Input: part model. Units: mm. Frame: model coordinates. A direction names the side the tool comes from. Round coordinates to 2 decimals unless told otherwise and drop trailing zeros. Loops run counter-clockwise (first coordinate to the right, second up) from the corner with the lowest first, then second, coordinate; pieces in that order, holes last. Notation, with made-up numbers: (88.25, -11.5) - (121.25, -11.5) arc R9 cw to (121.25, 0.5) - close; hole circle Ø11 at (18, 87.5). An arc over 180 degrees is marked (long way). One line per question, with ' | ' between items. Start each with the question number.
Item 1: Set-up query: faces 4 (the face through (34.925, -23, 0)), 5 (the face through (0, -39.37, 0)). Return all of +Z, -Z, +X, -X, +Y, -Y with unobstructed straight access to the full face (end or side cutting, diameter ignored); none if empty.
Item 2: Material intervals for line 1 along Y through (x, z) = (12, -3); line 2 along X through (y, z) = (-16, 11.75) (3 decimals), sorted ascending.
Item 3: Draft query along X for faces 1 (the face through (29.845, -22, 0)), 2 (the face through (-34.925, -22, 0)), 3 (the face through (0, -44.45, 0)). Return one class per face: pulls with the +X half, pulls with the -X half, needs draft (parallel to the pull), parting line crosses it, or undercut.
Item 4: Section A-A, the plane x = 20.5. Return loops of the section in (y, z), plus the area to 3 significant figures.
Item 5: Section C-C, the plane y = -23.5. Return loops of the section in (x, z) (3 decimals).
Item 6: Section B-B, the plane z = 9.75. Return loops of the section in (x, y) (3 decimals).
```python
from build123d import *

# Parameters (mm, degrees)
F0_W     = 69.85
F0_H     = 25.4
F1_DEPTH = 5.08
F2_W     = 39.37
F2_H     = 25.4
F3_DEPTH = 5.08
F4_W     = 64.77
F4_H     = 25.4
F5_DEPTH = 5.08
F6_W     = 39.37
F6_H     = 25.4
F7_DEPTH = 5.08


with BuildPart() as f1:
    # F0 (on Front) → F1 (new body)
    with BuildSketch(Plane.XZ):
        Rectangle(F0_W, F0_H)
    extrude(amount=F1_DEPTH)

    # F2 (on face) → F3 (join)
    with BuildSketch(Plane(origin=(-34.925, 0, 0), x_dir=(0, -1, 0), z_dir=(-1, 0, 0))):
        with Locations((24.765, 0)):
            Rectangle(F2_W, F2_H)
    extrude(amount=-F3_DEPTH)

    # F4 (on face) → F5 (join)
    with BuildSketch(Plane.XZ.offset(44.45)):
        with Locations((2.54, 0)):
            Rectangle(F4_W, F4_H)
    extrude(amount=-F5_DEPTH)

    # F6 (on face) → F7 (join)
    with BuildSketch(Plane.YZ.offset(34.925)):
        with Locations((-19.685, 0)):
            Rectangle(F6_W, F6_H)
    extrude(amount=-F7_DEPTH)


solid = f1.part
```
Return value:
1) face 4: +Z, -Z, +X, +Y, -Y | face 5: +Z, -Z
2) line 1: -44.45 to -39.37, -5.08 to 0 | line 2: -34.925 to -29.845, 29.845 to 34.925
3) face 1: undercut | face 2: pulls with the -X half | face 3: needs draft
4) outline: (-44.45, -12.7) - (-39.37, -12.7) - (-39.37, 12.7) - (-44.45, 12.7) - close; (-5.08, -12.7) - (0, -12.7) - (0, 12.7) - (-5.08, 12.7) - close | area: 258 mm2
5) outline: (-34.925, -12.7) - (-29.845, -12.7) - (-29.845, 12.7) - (-34.925, 12.7) - close; (29.845, -12.7) - (34.925, -12.7) - (34.925, 12.7) - (29.845, 12.7) - close
6) outline: (-34.925, -44.45) - (34.925, -44.45) - (34.925, 0) - (-34.925, 0) - close; hole (-29.845, -39.37) - (29.845, -39.37) - (29.845, -5.08) - (-29.845, -5.08) - close
